The drawing under review shows one solid part. Ordinate dimensions are in mm from its lowest x, y, z. A direction names the side the tool comes from. Round coordinates to 2 decimals unless told otherwise and drop trailing zeros. Loops run counter-clockwise (first coordinate to the right, second up) from the corner with the lowest first, then second, coordinate; pieces in that order, holes last. Notation, with made-up numbers: M 4.5,79 L 31.5,79 A23 ccw 31.5,117 Z; hole C 23,38 d4. An arc over 180 degrees is marked long. Use a Markdown table: item, result.
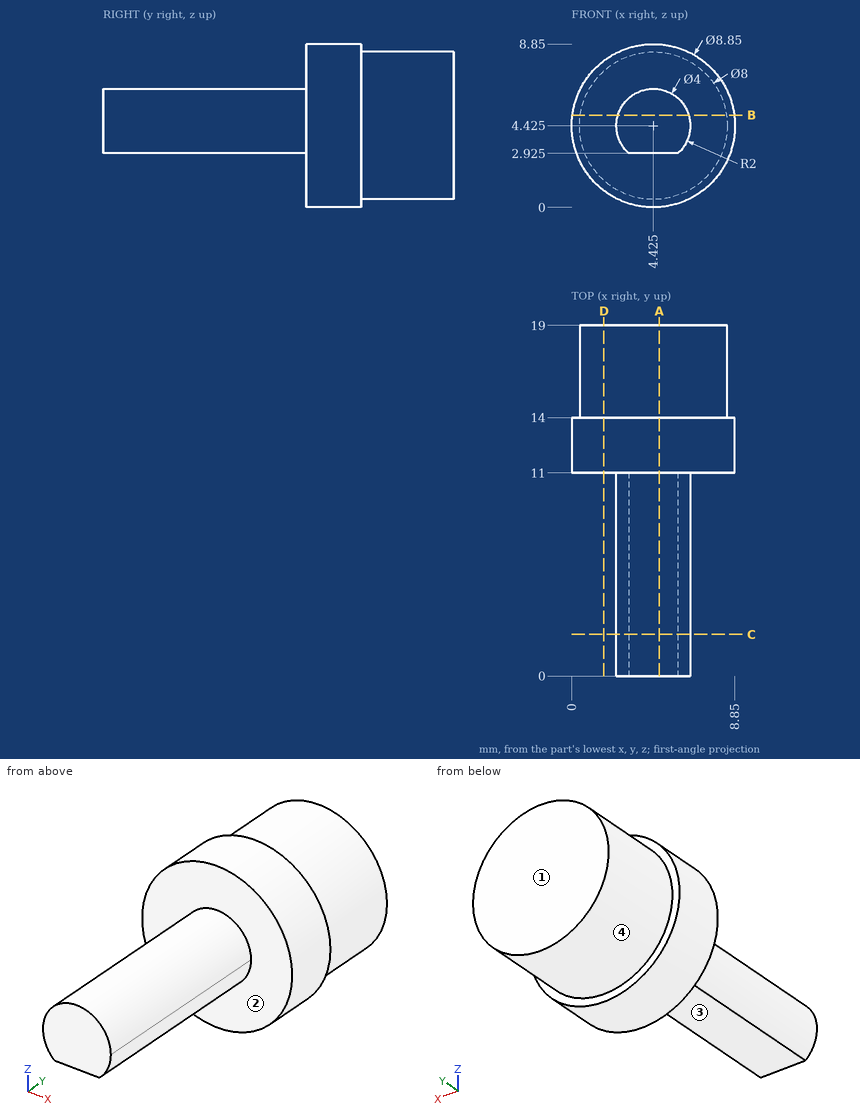
1. Machinability: for the marked faces 1, 2, 3 and 4, which of the approach directions +Z, -Z, +X, -X, +Y, -Y give a long, thin tool a straight path to every point of the face, cutting with its end or side? Answer none if there is none.
Check values:
| item | result |
|---|---|
| face 1 | +Z, -Z, +X, -X, +Y |
| face 2 | -Y |
| face 3 | -Z, +X, -X, -Y |
| face 4 | +Y |
2. Take a section at C-C on y = 2.25. Give the boundary of the cut face in (x, z) (3 decimals).
Check values:
| item | result |
|---|---|
| outline | M 3.102,2.925 L 5.748,2.925 A2 ccw long Z |
3. Take a section at B-B on z = 5. Give the boundary of the cut face in (x, y), and give its area (3 significant figures).
Check values:
| item | result |
|---|---|
| outline | M 0.04,11 L 2.51,11 L 2.51,0 L 6.34,0 L 6.34,11 L 8.81,11 L 8.81,14 L 8.38,14 L 8.38,19 L 0.47,19 L 0.47,14 L 0.04,14 Z |
| area | 108 mm² |
4. Take a section at A-A on x = 4.75. Give the boundary of the cut face in (y, z) (3 decimals), and give its area (3 significant figures).
Check values:
| item | result |
|---|---|
| outline | M 0,2.925 L 11,2.925 L 11,0.012 L 14,0.012 L 14,0.438 L 19,0.438 L 19,8.412 L 14,8.412 L 14,8.838 L 11,8.838 L 11,6.398 L 0,6.398 Z |
| area | 105 mm² |
5. Wall thickness on line 1 along Y through (x, z) = (7.75, 1.75); line 2 along Y through (x, z) = (2.25, 6.5); line 3 along X through (y, z) = (16.5, 1.25): over which ranges is each line inside the solid? List them lowest first. Write a range as from..to.
Check values:
| item | result |
|---|---|
| line 1 | y = 11..14 |
| line 2 | y = 11..19 |
| line 3 | x = 1.99..6.86 |
6. Take a section at D-D on x = 1.75. Give the boundary of the cut face in (y, z).
Check values:
| item | result |
|---|---|
| outline | M 11,0.9 L 14,0.9 L 14,1.45 L 19,1.45 L 19,7.4 L 14,7.4 L 14,7.95 L 11,7.95 Z |
7. Insertion check: pin 1 (1 mm diameter, centred on x = 5.5, z = 2.5, fed in from -Y); pin 2 (3 mm diameter, centred on x = 5, y = 9, fed in from -Z) (3 decimals); pin 3 (1.5 mm diameter, centred on x = 7, z = 1.5, fed in from -Y); pin 4 (4 mm diameter, centred on y = 11, z = 2, fed in from +X). Each pin has a flat end and moves straight along its axis. Give the tip position at first contact, or say it passes through.
Check values:
| item | result |
|---|---|
| pin 1 | stops at y = 0 |
| pin 2 | stops at z = 2.925 |
| pin 3 | stops at y = 11 |
| pin 4 | stops at x = 8.83 |
